Input: part model. Units: mm. Frame: model coordinates. A direction names the side the tool comes from. Coordinates: 2 decimals unless noted, no trailing zeros. Write each loop counter-clockwise with the first axis right and the second up, starting at its lowest first coordinate (ties: lowest second). Pieces come first, ordered by that corner, then holes. Notation, with made-up numbers: (26.5, 60.5) - (82.5, 60.5) arc R8 cw to (82.5, 73.5) - close; hole circle Ø1 at (13.25, -27.5). An arc over 180 degrees is marked (long way). Use a Markdown table: item, result. Add a question column.
Q1. Set-up query: faces 1 (the face through (2, -2, 3)), 2 (the face through (-1.5, 0.07, 1.61)). Return all of +Z, -Z, +X, -X, +Y, -Y with unobstructed straight access to the full face (end or side cutting, diameter ignored); none if empty.
Q2. Section query C-C (z = 0.4). Return the cut outline in (x, y), then the cut area to 3 significant figures.
Q3. Section query A-A (x = 0). Return the cut outline in (y, z).
Q4. Material intervals for probe 1 along Y at (x, z) = (0, 0.9); probe 2 along Z at (x, y) = (-6, 1.5); probe 3 along Y at (x, z) = (-0.75, 0.35), sorted ascending. Write a range as from..to.
from build123d import *

# Parameters (mm, degrees)
ESQUISSE1_R      = 8
ESQUISSE1_R_2    = 1.5
EXTRUSION1_DEPTH = 3
ESQUISSE2_R      = 2
ESQUISSE2_R_2    = 1.5
EXTRUSION2_DEPTH = 0.25
CONG_1_R         = 0.2


with BuildPart() as part:
    # Esquisse1 → Extrusion1 (new body)
    with BuildSketch(Plane.XY):
        Circle(ESQUISSE1_R)
        Circle(ESQUISSE1_R_2, mode=Mode.SUBTRACT)
    extrude(amount=EXTRUSION1_DEPTH)

    # Esquisse2 → Extrusion2 (add)
    with BuildSketch(Plane.XY.offset(3)):
        Circle(ESQUISSE2_R)
        Circle(ESQUISSE2_R_2, mode=Mode.SUBTRACT)
    extrude(amount=EXTRUSION2_DEPTH)

    # Congé1
    cong_1_edges = [part.edges().sort_by_distance(p)[0] for p in [
        (-8, 0, 0),
        (-8, 0, 3),
        (-2, 0, 3),
        (-1.5, 0, 3.25),
        (-1.5, 0, 0),
    ]]
    fillet(cong_1_edges, radius=CONG_1_R)


solid = part.part
Values follow:
| question | item | result |
|---|---|---|
| 1 | face 1 | +Z |
| 1 | face 2 | +Z, -Z |
| 2 | outline | circle Ø16 at (0, 0); hole circle Ø3 at (0, 0) |
| 2 | area | 194 mm2 |
| 3 | outline | (-8, 0.2) arc R0.2 ccw to (-7.8, 0) - (-1.7, 0) arc R0.2 ccw to (-1.5, 0.2) - (-1.5, 3.05) arc R0.2 ccw to (-1.7, 3.25) - (-2, 3.25) - (-2, 3.2) arc R0.2 cw to (-2.2, 3) - (-7.8, 3) arc R0.2 ccw to (-8, 2.8) - close; (1.5, 0.2) arc R0.2 ccw to (1.7, 0) - (7.8, 0) arc R0.2 ccw to (8, 0.2) - (8, 2.8) arc R0.2 ccw to (7.8, 3) - (2.2, 3) arc R0.2 cw to (2, 3.2) - (2, 3.25) - (1.7, 3.25) arc R0.2 ccw to (1.5, 3.05) - close |
| 4 | probe 1 | -8..-1.5, 1.5..8 |
| 4 | probe 2 | 0..3 |
| 4 | probe 3 | -7.96..-1.3, 1.3..7.96 |
